Check sheet for the modelled part. Datum: model origin and axes. Units: mm. Face numbers are marked on the shaded views. A direction names the side the tool comes from. Round coordinates to 2 decimals unless told otherwise and drop trailing zeros. Write each loop counter-clockwise with the first axis right and the second up, starting at its lowest first coordinate (ties: lowest second). Pieces come first, ordered by that corner, then holes. Notation, with made-up numbers: (-25, 56) -> (28, 56) arc R26 ccw to (28, 91) -> close; hole circle Ø3 at (24.5, 38). An arc over 180 degrees is marked (long way). Put each result on its own line as item: value. Start each with the question number.
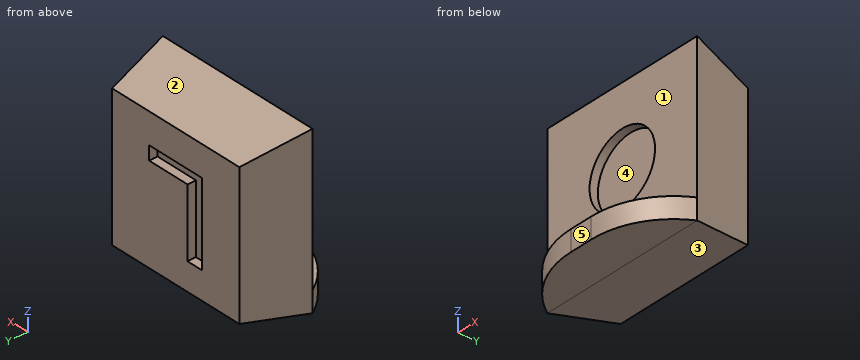
from build123d import *

# Parameters (mm, degrees)
SKETCH1_W               = 8
SKETCH1_H               = 8
BOSS_EXTRUDE1_DEPTH     = 3
CUT_EXTRUDE1_DEPTH      = 12.704699911
CUT_EXTRUDE1_DEPTH_BACK = 12.704699911
CUT_EXTRUDE2_DEPTH      = 11
SKETCH4_R               = 1.75
CUT_EXTRUDE3_DEPTH      = 0.4
SKETCH5_W               = 8
SKETCH5_H               = 1
BOSS_EXTRUDE2_DEPTH     = 2
FILLET1_R               = 4
CUT_EXTRUDE4_DEPTH      = 0.4


with BuildPart() as part:
    # Sketch1 → Boss-Extrude1 (new body)
    with BuildSketch(Plane(origin=(0, 0, 0), x_dir=(1, 0, 0), z_dir=(0, 1, 0))):
        with Locations((4, 4)):
            Rectangle(SKETCH1_W, SKETCH1_H)
    extrude(amount=BOSS_EXTRUDE1_DEPTH)

    # Sketch2 → Cut-Extrude1 (cut, two sides: drawn at the far end of the back side and taken through both)
    with BuildSketch(Plane.XY.offset(-CUT_EXTRUDE1_DEPTH_BACK)):
        Polygon((0, 0), (0.6, 3), (0, 3), align=None)
        Polygon((8, 0), (7.4, 3), (8, 3), align=None)
    extrude(amount=CUT_EXTRUDE1_DEPTH + CUT_EXTRUDE1_DEPTH_BACK, mode=Mode.SUBTRACT)

    # Sketch3 → Cut-Extrude2 (cut)
    with BuildSketch(Plane(origin=(0, 0, 0), x_dir=(0, 0, -1), z_dir=(1, 0, 0))):
        Polygon((0, 0), (0.6, 3), (0, 3), align=None)
        Polygon((8, 3), (7.4, 3), (8, 0), align=None)
    extrude(amount=CUT_EXTRUDE2_DEPTH, mode=Mode.SUBTRACT)

    # Sketch4 → Cut-Extrude3 (cut)
    with BuildSketch(Plane.XZ):
        with Locations(Location((4, -3.75, 0), (0, 0, 270))):
            Circle(SKETCH4_R)
    extrude(amount=-CUT_EXTRUDE3_DEPTH, mode=Mode.SUBTRACT)

    # Sketch5 → Boss-Extrude2 (add)
    with BuildSketch(Plane.XZ):
        with Locations((4, -7.5)):
            Rectangle(SKETCH5_W, SKETCH5_H)
    extrude(amount=BOSS_EXTRUDE2_DEPTH)

    # Fillet1
    # the kernel refuses this fillet: 4 mm, written as the material it takes off along each edge
    with BuildSketch(Plane(origin=(8, -2, -16.660254038), x_dir=(0, 1, 0), z_dir=(0, 0, 1)), Plane(origin=(0, -2, 1.660254038), x_dir=(0, 1, 0), z_dir=(0, 0, -1))) as fillet1_piece_1:
        with BuildLine():
            CenterArc((4, 3.464101615), FILLET1_R, 180, 60)
            Line((0, 3.464101615), (-0.08, 3.464101615))
            Line((-0.08, 3.464101615), (-0.08, 0))
            Line((-0.08, 0), (0, -0.08))
            ThreePointArc((0, -0.08), (1, -0.08), (1.96, -0.069282032))
            Line((1.96, -0.069282032), (2, 0))
        make_face()
    extrude(amount=18.320508076, mode=Mode.SUBTRACT)

    # Sketch6 → Cut-Extrude4 (cut)
    with BuildSketch(Plane(origin=(0, 3, 0), x_dir=(1, 0, 0), z_dir=(0, 1, 0))):
        Polygon((2.598201218, 2.07225421), (2.598201218, 6.07225421), (3.367431987, 6.07225421), (3.367431987, 2.738920877), (5.418714038, 2.738920877), (5.418714038, 2.07225421), align=None)
    extrude(amount=-CUT_EXTRUDE4_DEPTH, mode=Mode.SUBTRACT)


solid = part.part
1. Section check D-D, the plane x = 4. Enter the section's corners in (y, z).
2. Access from +Z, -Z, +X, -X, +Y, -Y to the whole of each face (thin tool, end or side, straight path). Record for the marked faces 1 and 2.
3. Draft check along Z on the marked faces 3, 4 and 5. Enter one of: released by +Z, released by -Z, zero draft, split by the parting line, or undercut.
4. Material ranges on L1, parallel to Y at x = 3, z = -0.75; L2, parallel to Z at x = 3, y = 0.1; L3, parallel to X at y = 0.2, z = -3.75, recorded low to high. Write a range as [from, to].
5. Section check B-B, the plane x = 6.25. Enter the section's corners in (y, z).
6. Section check C-C, the plane y = 1.2. Enter the section's corners in (x, z), then the cut area to 3 significant figures.
7. Gauge pin test, flat ends, axial feed: P1, Ø1.6, axis at x = 3, y = -1.5, coming from the +Z side; P2, Ø1, axis at x = 6.5, z = -1, coming from the -Y side; P3, Ø1, axis at y = 2, z = -4.5, coming from the +X side. Record the tip position at first contact, or that the pin passes through.
8. Section check A-A, the plane z = -3.75. Enter the section's corners in (x, y), then the cut area to 3 significant figures.
Reply:
1. outline: (-2, -8) -> (0, -8) -> (3, -7.4) -> (3, -2.74) -> (2.6, -2.74) -> (2.6, -2.07) -> (3, -2.07) -> (3, -0.6) -> (0, 0) -> (0, -2) -> (0.4, -2) -> (0.4, -5.5) -> (0, -5.5) -> (0, -7) -> (-2, -7) -> close
2. face 1: +Z, +X, -X, -Y
2. face 2: +Z, +X, -X, +Y
3. face 3: released by -Z
3. face 4: undercut
3. face 5: zero draft
4. L1: y = [0, 3]
4. L2: z = [-7.98, -5.19], [-2.31, -0.02]
4. L3: x = [0.04, 2.25], [5.75, 7.96]
5. outline: (-1.61, -8) -> (0, -8) -> (3, -7.4) -> (3, -0.6) -> (0, 0) -> (0, -7) -> (-1.61, -7) -> close
6. outline: (0.24, -7.76) -> (7.76, -7.76) -> (7.76, -0.24) -> (0.24, -0.24) -> close
6. area: 56.6 mm2
7. P1: stops at z = -7
7. P2: stops at y = 0
7. P3: stops at x = 7.7
8. outline: (0, 0) -> (2.25, 0) -> (2.25, 0.4) -> (5.75, 0.4) -> (5.75, 0) -> (8, 0) -> (7.4, 3) -> (3.37, 3) -> (3.37, 2.6) -> (2.6, 2.6) -> (2.6, 3) -> (0.6, 3) -> close
8. area: 20.5 mm2
